Source: CAD feature listing. Evaluate the final solid. Frame: model axes, mm. A direction names the side the tool comes from. Round coordinates to 2 decimals unless told otherwise and drop trailing zeros. Write each loop counter-clockwise with the first axis right and the second up, starting at its lowest first coordinate (ties: lowest second). Pieces come first, ordered by that corner, then holes. Notation, with made-up numbers: M -14,32.5 L 15,32.5 A30 cw 15,69.5 Z; hole C -3,53.25 d2. An arc over 180 degrees is marked long. Put each result on its own line as item: value. Start each with the question number.
```python
from build123d import *

# Parameters (mm, degrees)
F1_DEPTH = 17
F2_T     = -3
F3_R     = 4
F4_DEPTH = 5
F5_R     = 0.49999
F6_SIZE  = 0.5


# Not quite as in the source:
# - a fillet or chamfer is up to 0.001 mm smaller than in the source, because OpenCascade refuses the exact size


with BuildPart() as f1:
    # F0 (on Top) → F1 (new body)
    with BuildSketch(Plane.XY):
        with BuildLine():
            ThreePointArc((-20.5, -3), (-18.7426406871, -7.2426406871), (-14.5, -9))
            Line((-14.5, -9), (14.5, -9))
            ThreePointArc((14.5, -9), (18.7426406871, -7.2426406871), (20.5, -3))
            Line((20.5, -3), (20.5, 3))
            ThreePointArc((20.5, 3), (18.7426406871, 7.2426406871), (14.5, 9))
            Line((14.5, 9), (-14.5, 9))
            ThreePointArc((-14.5, 9), (-18.7426406871, 7.2426406871), (-20.5, 3))
            Line((-20.5, 3), (-20.5, -3))
        make_face()
    extrude(amount=F1_DEPTH)

    # F2
    f2_openings = [f1.faces().sort_by_distance(p)[0] for p in [
        (0, 0, 17),
        (0, 0, 0),
    ]]
    offset(amount=F2_T, openings=f2_openings)

    # F3 (on face) → F4 (cut)
    with BuildSketch(Plane.XZ.offset(9)):
        with Locations((-10, 8.5)):
            Circle(F3_R)
        with Locations((10, 8.5)):
            Circle(F3_R)
    extrude(amount=-F4_DEPTH, mode=Mode.SUBTRACT)

    # F5 (radius 0.5 in the source; OpenCascade refuses exactly that, so slightly less here)
    f5_edges = [f1.edges().sort_by_distance(p)[0] for p in [
        (0, 9, 0),
        (0, -6, 0),
        (6, -9, 8.5),
        (-14, -9, 8.5),
    ]]
    fillet(f5_edges, radius=F5_R)

    # F6
    f6_edges = [f1.edges().sort_by_distance(p)[0] for p in [
        (0, -9, 17),
        (0, -6, 17),
    ]]
    chamfer(f6_edges, length=F6_SIZE)


solid = f1.part
```
(1) Ray query, line 1 along Y through (x, z) = (-14.5, 15.25); line 2 along X through (y, z) = (2, 16); line 3 along Z through (x, y) = (10, -7.3). Return the intervals inside material, ascending.
(2) Access query for faces 4 (the cylindrical face through (-18.696, 7.289, 8.388)), 5 (the conical face through (16.741, 5.193, 16.635)), 6 (the flat face through (-17.5, 0, 8)), 7 (the cylindrical face through (6.004, -7.268, 8.676)). Directions: +Z, -Z, +X, -X, +Y, -Y. A direction counts if a zero-diameter tool reaches every point of the face in a straight line with its end or side. Return the directions, or none.
(3) Section query A-A (y = -2.25). Return loops of the section in (x, z).
(4) Section query C-C (x = 10). Return loops of the section in (y, z), and give its area (3 significant figures).
(5) Contact query for a flat-ended pin moving along its axis: P1, Ø10, axis at y = -5.5, z = 5.5, coming from the +X side. Output: stop coordinate, or through.
(6) Pull-direction query (X, two-part tool) for faces 1 (the conical face through (-16.693, 5.241, 16.635)), 2 (the conical face through (18.533, 6.946, 16.858)), 3 (the cylindrical face through (-18.789, -7.196, 8.388)); classes: +X half, -X half, draft (parallel to the pull), parting line (faces both ways), or undercut.
(7) Section query B-B (x = -1.5). Return loops of the section in (y, z).
Entries:
1. line 1: -9 to -6, 6 to 9
1. line 2: -20.5 to -17.5, 17.5 to 20.5
1. line 3: 0 to 4.5, 12.5 to 17
2. face 4: +Z, -Z, -X, +Y
2. face 5: +Z
2. face 6: +Z, -Z
2. face 7: -Y
3. outline: M -20.5,0.5 A0.5 ccw -20,0 L -18,0 A0.5 ccw -17.5,0.5 L -17.5,16.5 L -18,17 L -20,17 L -20.5,16.5 Z; M 17.5,0.5 A0.5 ccw 18,0 L 20,0 A0.5 ccw 20.5,0.5 L 20.5,16.5 L 20,17 L 18,17 L 17.5,16.5 Z
4. outline: M -9,0.5 A0.5 ccw -8.5,0 L -6.5,0 A0.5 ccw -6,0.5 L -6,4.5 L -8.5,4.5 A0.5 ccw -9,4 Z; M -9,13 A0.5 ccw -8.5,12.5 L -6,12.5 L -6,16.5 L -6.5,17 L -8.5,17 L -9,16.5 Z; M 6,0.5 A0.5 ccw 6.5,0 L 8.5,0 A0.5 ccw 9,0.5 L 9,16.5 L 8.5,17 L 6.5,17 L 6,16.5 Z
4. area: 77.2 mm2
5. P1: x = 20.5
6. face 1: undercut
6. face 2: +X half
6. face 3: -X half
7. outline: M -9,0.5 A0.5 ccw -8.5,0 L -6.5,0 A0.5 ccw -6,0.5 L -6,16.5 L -6.5,17 L -8.5,17 L -9,16.5 Z; M 6,0.5 A0.5 ccw 6.5,0 L 8.5,0 A0.5 ccw 9,0.5 L 9,16.5 L 8.5,17 L 6.5,17 L 6,16.5 Z
